Build history of the part. All positions in model axes, mm. Face numbers are marked on the shaded views. A direction names the side the tool comes from. Round coordinates to 2 decimals unless told otherwise and drop trailing zeros. Loops run counter-clockwise (first coordinate to the right, second up) from the corner with the lowest first, then second, coordinate; pieces in that order, holes last. Notation, with made-up numbers: M 45,52.5 L 73,52.5 A25 cw 73,75.5 Z; hole C -14.75,-32 d8. An arc over 180 degrees is marked long. One line per item, written item: value.
```python
from build123d import *

# Parameters (mm, degrees)
F0_W      = 20
F0_H      = 70
F1_DEPTH  = 30
F2_W      = 30
F2_H      = 10
F3_DEPTH  = 10
F4_R      = 2.05
F5_DEPTH  = 10
F6_W      = 11
F6_H      = 30
F7_DEPTH  = 50
F9_DEPTH  = 5
F10_SIZE2 = 10.99999
F10_SIZE  = 49.99999
F11_W     = 30
F11_H     = 55
F12_DEPTH = 0.5


# Not quite as in the source:
# - a fillet or chamfer is up to 0.001 mm smaller than in the source, because OpenCascade refuses the exact size


with BuildPart() as f1:
    # F0 (on Front) → F1 (new body)
    with BuildSketch(Plane.XZ):
        with Locations((-10, 35)):
            Rectangle(F0_W, F0_H)
    extrude(amount=F1_DEPTH)

    # F2 (on face) → F3 (cut)
    with BuildSketch(Plane(origin=(-20, 0, 0), x_dir=(0, -1, 0), z_dir=(-1, 0, 0))):
        with Locations((15, 5)):
            Rectangle(F2_W, F2_H)
    extrude(amount=-F3_DEPTH, mode=Mode.SUBTRACT)

    # F4 (on face) → F5 (cut, through all)
    with BuildSketch(Plane(origin=(-10, 0, 0), x_dir=(0, -1, 0), z_dir=(-1, 0, 0))):
        with Locations((5, 5)):
            Circle(F4_R)
        with Locations((25, 5)):
            Circle(F4_R)
    extrude(amount=-F5_DEPTH, mode=Mode.SUBTRACT)

    # F6 (on face) → F7 (cut)
    with BuildSketch(Plane.XY.offset(70)):
        with Locations((-5.5, -15)):
            Rectangle(F6_W, F6_H)
    extrude(amount=-F7_DEPTH, mode=Mode.SUBTRACT)

    # F8 (on face) → F9 (join)
    with BuildSketch(Plane.XY.offset(70)):
        with BuildLine():
            ThreePointArc((-17, -11.0388736054), (-19.25, -7), (-17, -2.9611263946))
            Line((-17, -2.9611263946), (-17, 0))
            Line((-17, 0), (-20, 0))
            Line((-20, 0), (-20, -30))
            Line((-20, -30), (-17, -30))
            Line((-17, -30), (-17, -27.0388736054))
            ThreePointArc((-17, -27.0388736054), (-19.25, -23), (-17, -18.9611263946))
            Line((-17, -18.9611263946), (-17, -11.0388736054))
        make_face()
    extrude(amount=F9_DEPTH)

    # F10 (size 50 and 11 in the source; OpenCascade refuses exactly that, so slightly less here)
    f10_edges = [f1.edges().sort_by_distance(p)[0] for p in [
        (-11, -15, 20),
    ]]
    f10_side = f1.faces().sort_by_distance((-11, -15, 45))[0]
    chamfer(f10_edges, length=F10_SIZE, length2=F10_SIZE2, reference=f10_side)

    # F11 (on face) → F12 (cut)
    with BuildSketch(Plane(origin=(-20, 0, 0), x_dir=(0, -1, 0), z_dir=(-1, 0, 0))):
        with Locations((15, 37.5)):
            Rectangle(F11_W, F11_H)
    extrude(amount=-F12_DEPTH, mode=Mode.SUBTRACT)


solid = f1.part
```
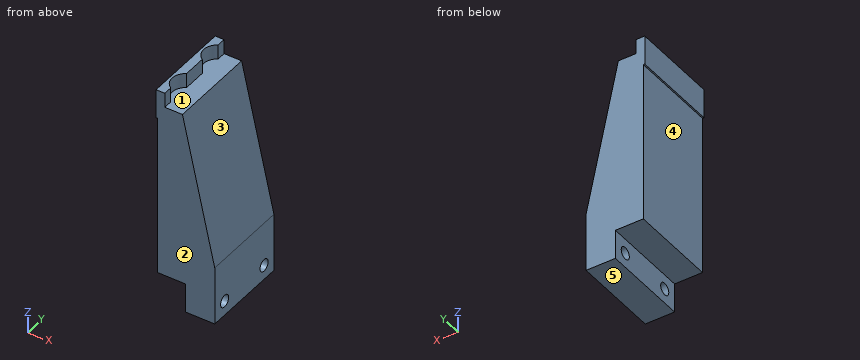
Item 1: Pull direction Y, two halves, no side cores. Call the marked faces 1, 2 and 3: pulls with the +Y half, pulls with the -Y half, needs draft (parallel to the pull), parting line crosses it, or undercut.
Check values:
face 1: undercut
face 2: pulls with the -Y half
face 3: needs draft
Item 2: Slice it at A-A, the plane z = 5. Give the cut face in (x, y).
Check values:
outline: M -10,-30 L 0,-30 L 0,-27.05 L -10,-27.05 Z; M -10,-22.95 L 0,-22.95 L 0,-7.05 L -10,-7.05 Z; M -10,-2.95 L 0,-2.95 L 0,0 L -10,0 Z
Item 3: Slice it at C-C, the plane x = -5. Give the cut face in (y, z).
Check values:
outline: M -30,0 L 0,0 L 0,42.73 L -30,42.73 Z; hole C -25,5 d4.1; hole C -5,5 d4.1
Item 4: Wall check: line 1 along X through (y, z) = (-3.25, 9.5); line 2 along X through (y, z) = (-21, 18.5); line 3 along Z through (x, y) = (-13, -27). Give the ranges that are in metal, low to high.
Check values:
line 1: x = -10 to 0
line 2: x = -19.5 to 0
line 3: z = 10 to 70
Item 5: Which spindle directions (+Z, -Z, +X, -X, +Y, -Y) get a long thin tool onto all of the face, cutting with end or side? Do the marked faces 4 and 5. Say none if no direction does.
Check values:
face 4: -Z, -X, +Y, -Y
face 5: -Z, +X, -X, +Y, -Y
Item 6: Drop flat-ended pins along their axis: P1, Ø1.5, axis at x = -5, z = 52, coming from the -Y side; P2, Ø2.5, axis at x = -14.5, y = -9.5, coming from the +Z side; P3, Ø9, axis at y = -11.5, z = 27, coming from the -X side; P4, Ø5, axis at y = -18.5, z = 5, coming from the -X side. Give the stop position or say it passes through.
Check values:
P1: passes through
P2: stops at z = 70
P3: stops at x = -19.5
P4: stops at x = -10
